from build123d import *

# Parameters (mm, degrees)
F0_W     = 575
F0_H     = 300
F1_DEPTH = 50
F2_W     = 50
F2_H     = 300
F3_DEPTH = 450
F5_DEPTH = 50
F8_W     = 500
F8_H     = 125
F9_DEPTH = 1150.001


# Not quite as in the source:
# - a feature of the source that left no trace in its solid (it failed there, or was rolled back) is left out


with BuildPart() as f1:
    # F0 (on Top) → F1 (new body)
    with BuildSketch(Plane.XY):
        with Locations((287.5, -150)):
            Rectangle(F0_W, F0_H)
    extrude(amount=-F1_DEPTH)

    # F2 (on face) → F3 (join)
    with BuildSketch(Plane(origin=(0, 0, -50), x_dir=(1, 0, 0), z_dir=(0, 0, -1))):
        with Locations((550, 150)):
            Rectangle(F2_W, F2_H)
    extrude(amount=F3_DEPTH)

    # F4 (on face) → F5 (join, through all)
    with BuildSketch(Plane.YZ.offset(575)):
        Polygon((50, -30), (0, -80), (0, -150.7106781187), (120.7106781187, -30), align=None)
    extrude(amount=-F5_DEPTH)

    # F6: F1 across plane


with BuildPart() as f1_1:
    add(f1.part)
    add(f1.part.mirror(Plane.YZ))

    # F7: F1 across plane


with BuildPart() as f1_2:
    add(f1_1.part)
    add(f1_1.part.mirror(Plane.XZ))

    # F8 (on face) → F9 (cut, through all)
    with BuildSketch(Plane.YZ.offset(575)):
        with Locations((0, -112.5)):
            Rectangle(F8_W, F8_H)
    extrude(amount=-F9_DEPTH, mode=Mode.SUBTRACT)


solid = f1_2.part
Source: CAD feature listing. Evaluate the final solid. Frame: model axes, mm. A direction names the side the tool comes from. Give positions to 0.01 mm unless a question says otherwise; leave off trailing zeros. Write each loop counter-clockwise with the first axis right and the second up, starting at its lowest first coordinate (ties: lowest second). Pieces come first, ordered by that corner, then holes. Notation, with made-up numbers: (-31, 21) - (-10, 21) arc R26 cw to (-10, 53) - close; hole circle Ø11 at (-14, -8.5). An arc over 180 degrees is marked (long way). Write item = value, one per line. Start each with the question number.
Q1. Cut plane C-C, the plane z = -280.5. Return loops of the section in (x, y).
Q2. Cut plane D-D, the plane x = 290. Return loops of the section in (y, z).
Q3. Reachability of faces 5 (the flat face through (-550, -3, -175)), 6 (the flat face through (3, -300, -45)), 7 (the flat face through (525, -4, -322)) from +Z, -Z, +X, -X, +Y, -Y: full face, straight path, thin tool, end or side. Return the list, or none.
Q4. Cut plane B-B, the plane y = 118. Return loops of the section in (x, z).
Q5. Cut plane A-A, the plane z = -86.5. Return loops of the section in (x, y).
Q6. Draft query along Y for faces 1 (the flat face through (550, 250, -113)), 2 (the flat face through (3, 300, -45)), 3 (the flat face through (550, -250, -113)), 4 (the flat face through (-575, -4, -302)). Return one class per face: +Y half, -Y half, draft (parallel to the pull), parting line (faces both ways), or undercut.
Q7. Material intervals for probe 1 along X at (y, z) = (-22, -355.5); probe 2 along Z at (x, y) = (-87, -201), sorted ascending.
Q8. Pin query (flat end, axial travel): pin 1 Ø12 at (x, y) = (-334.5, -124) entering from -Z. Return the tip coordinate at first contact, or that it passes through.
Computed values:
q1.outline = (-575, -300) - (-525, -300) - (-525, 300) - (-575, 300) - close; (525, -300) - (575, -300) - (575, 300) - (525, 300) - close
q2.outline = (-300, -50) - (300, -50) - (300, 0) - (-300, 0) - close
q3.face_5 = +X, -X
q3.face_6 = +Z, -Z, +X, -X, -Y
q3.face_7 = -Z, +Y, -Y
q4.outline = (-575, -500) - (-525, -500) - (-525, -175) - (-575, -175) - close; (-575, -50) - (575, -50) - (575, 0) - (-575, 0) - close; (525, -500) - (575, -500) - (575, -175) - (525, -175) - close
q5.outline = (-575, -300) - (-525, -300) - (-525, -250) - (-575, -250) - close; (-575, 250) - (-525, 250) - (-525, 300) - (-575, 300) - close; (525, -300) - (575, -300) - (575, -250) - (525, -250) - close; (525, 250) - (575, 250) - (575, 300) - (525, 300) - close
q6.face_1 = undercut
q6.face_2 = +Y half
q6.face_3 = undercut
q6.face_4 = draft
q7.probe_1 = -575 to -525, 525 to 575
q7.probe_2 = -50 to 0
q8.pin_1 = -50
